Model file for the job. Use its own axes, mm. Face numbers are marked on the shaded views. A direction names the side the tool comes from. Round coordinates to 2 decimals unless told otherwise and drop trailing zeros. Loops run counter-clockwise (first coordinate to the right, second up) from the corner with the lowest first, then second, coordinate; pieces in that order, holes last. Notation, with made-up numbers: M 43,70.5 L 82,70.5 A12 ccw 82,80.5 Z; hole C 6.25,86 d3. An arc over 180 degrees is marked long. Use a Markdown table: item, result. Add a question column.
Q1. Cut at D-D (x = 12.5). Give the cut face in (y, z).
Q2. Probe line 1 (Y direction, x = 1, z = -0.5); line 2 (Z direction, x = 34, y = 28.5); line 3 (Z direction, x = -7, y = 16). List the from-to ranges inside material, lowest first. Write a range as from..to.
Q3. Pin check, flat tips, straight feed: pin 1 (7 mm diameter, centred on x = 45, y = 0, fed in from +Z); pin 2 (10.5 mm diameter, centred on x = 0, y = 45, fed in from -Z); pin 3 (12 mm diameter, centred on y = 6.5, z = -11.5, fed in from +X); pin 4 (5 mm diameter, centred on x = -31, y = -13, fed in from +Z). Stop position of each tip, or through.
Q4. Mould opens along X. For the marked faces 1, 2 and 3 say: +X half, -X half, draft (parallel to the pull), parting line (faces both ways), or undercut.
Q5. Tool access for the marked faces 4 and 5: list every direction of +Z, -Z, +X, -X, +Y, -Y with a clear straight run to the whole face (end or side of a thin tool).
Q6. Cut at A-A (x = -45). Give the cut face in (y, z).
Q7. Cut at C-C (z = -4.5). Give the cut face in (x, y).
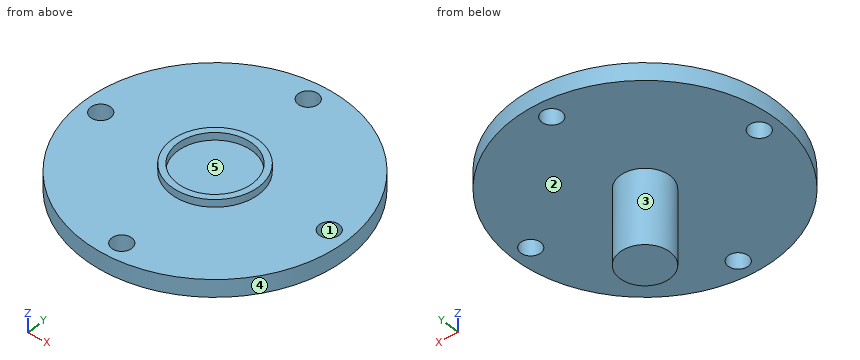
Autodesk Inventor part; units mm, degrees
ref_plane "YZ Plane" through (0, 0, 0) normal (1, 0, 0) x (0, 1, 0)
ref_plane "XZ Plane" through (0, 0, 0) normal (0, 1, 0) x (-1, 0, 0)
ref_plane "XY Plane" through (0, 0, 0) normal (0, 0, 1) x (1, 0, 0)
sketch "Sketch1" plane through (0, 0, 0) normal (0, 0, 1) x (1, 0, 0)
  circle A0 centre (0, 0) radius 52.5
  dimension "d0" = 105
extrude "Extrusion1" add sketch "Sketch1" against normal blind 7
sketch "Sketch2" plane through (0, 0, 0) normal (0, 0, 1) x (1, 0, 0)
  circle A0 centre (0, 0) radius 45 construction
  line L0 (0, 0) -> (0, 45) construction
  dimension "d3" = 90
hole "Hole1" at (0, 45, 0) direction (0, 0, -1) diameter 8 depth 7
pattern_circular "Circular Pattern1" count 4 over 360 about axis through (0, 0, -10) along (0, 0, 1) of "Hole1"
sketch "Sketch3" plane through (0, 0, -7) normal (0, 0, -1) x (-1, 0, 0)
  circle A0 centre (0, 0) radius 10
  dimension "d14" = 20
extrude "Extrusion2" add sketch "Sketch3" along normal blind 30
sketch "Sketch4" plane through (0, 0, 0) normal (0, 0, 1) x (1, 0, 0)
  circle A0 centre (0, 0) radius 15
  circle A1 centre (0, 0) radius 17.5
  dimension "d17" = 35
  dimension "d18" = 30
extrude "Extrusion3" add sketch "Sketch4" along normal blind 3
properties part number "Diff_Driveshaft_Output_V1"
Checked values:
| question | item | result |
|---|---|---|
| 1 | outline | M -50.99,-7 L 50.99,-7 L 50.99,0 L 12.25,0 L 12.25,3 L 8.29,3 L 8.29,0 L -8.29,0 L -8.29,3 L -12.25,3 L -12.25,0 L -50.99,0 Z |
| 2 | line 1 | y = -52.49..-48.87, -41.13..41.13, 48.87..52.49 |
| 2 | line 2 | z = -7..0 |
| 2 | line 3 | z = -7..3 |
| 3 | pin 1 | passes through |
| 3 | pin 2 | stops at z = -7 |
| 3 | pin 3 | stops at x = 52.44 |
| 3 | pin 4 | stops at z = 0 |
| 4 | face 1 | undercut |
| 4 | face 2 | draft |
| 4 | face 3 | parting line |
| 5 | face 4 | +Z, -Z |
| 5 | face 5 | +Z |
| 6 | outline | M -27.04,-7 L -4,-7 L -4,0 L -27.04,0 Z; M 4,-7 L 27.04,-7 L 27.04,0 L 4,0 Z |
| 7 | outline | C 0,0 d105; hole C -45,0 d8; hole C 0,-45 d8; hole C 0,45 d8; hole C 45,0 d8 |
